```python
from build123d import *

# Parameters (mm, degrees)
BOSS_EXTRUDE1_DEPTH     = 42
CUT_EXTRUDE1_DEPTH      = 51.635955605
CUT_EXTRUDE1_DEPTH_BACK = 51.635955605
SKETCH2_R               = 1.125
CHAMFER1_SIZE           = 12
CHAMFER1_SIZE2          = 2.115923769
CHAMFER2_SIZE           = 12
CHAMFER2_SIZE2          = 2.115923769


with BuildPart() as part:
    # Sketch1 → Boss-Extrude1 (new body)
    with BuildSketch(Plane.XY):
        Polygon((0, 0), (0, 20), (4, 20), (4, 4), (20, 4), (20, 0), align=None)
    extrude(amount=BOSS_EXTRUDE1_DEPTH)

    # Sketch2 → Cut-Extrude1 (cut, two sides: drawn at the far end of the back side and taken through both)
    with BuildSketch(Plane(origin=(0, 0, 0), x_dir=(0, 0, -1), z_dir=(0.7071067811865475, -0.7071067811865477, 0)).offset(-CUT_EXTRUDE1_DEPTH_BACK)):
        with Locations(Location((-40, 2.828427125, 0), (0, 0, 90))):
            Circle(SKETCH2_R)
        with Locations(Location((-37.285714286, 2.828427125, 0), (0, 0, 90))):
            Circle(SKETCH2_R)
        with Locations(Location((-34.571428571, 2.828427125, 0), (0, 0, 90))):
            Circle(SKETCH2_R)
        with Locations(Location((-31.857142857, 2.828427125, 0), (0, 0, 90))):
            Circle(SKETCH2_R)
        with Locations(Location((-29.142857143, 2.828427125, 0), (0, 0, 90))):
            Circle(SKETCH2_R)
        with Locations(Location((-26.428571429, 2.828427125, 0), (0, 0, 90))):
            Circle(SKETCH2_R)
        with Locations(Location((-23.714285714, 2.828427125, 0), (0, 0, 90))):
            Circle(SKETCH2_R)
        with Locations(Location((-21, 2.828427125, 0), (0, 0, 90))):
            Circle(SKETCH2_R)
        with Locations(Location((-18.285714286, 2.828427125, 0), (0, 0, 90))):
            Circle(SKETCH2_R)
        with Locations(Location((-15.571428571, 2.828427125, 0), (0, 0, 90))):
            Circle(SKETCH2_R)
        with Locations(Location((-12.857142857, 2.828427125, 0), (0, 0, 90))):
            Circle(SKETCH2_R)
        with Locations(Location((-10.142857143, 2.828427125, 0), (0, 0, 90))):
            Circle(SKETCH2_R)
        with Locations(Location((-7.428571429, 2.828427125, 0), (0, 0, 90))):
            Circle(SKETCH2_R)
        with Locations(Location((-4.714285714, 2.828427125, 0), (0, 0, 90))):
            Circle(SKETCH2_R)
        with Locations(Location((-2, 2.828427125, 0), (0, 0, 90))):
            Circle(SKETCH2_R)
    extrude(amount=CUT_EXTRUDE1_DEPTH + CUT_EXTRUDE1_DEPTH_BACK, mode=Mode.SUBTRACT)

    # Chamfer1
    chamfer1_edges = [part.edges().sort_by_distance(p)[0] for p in [
        (20, 0, 21),
    ]]
    chamfer1_side = [part.faces().sort_by_distance(p)[0] for p in [
        (10.669713524, 0, 21),
    ]]
    chamfer(chamfer1_edges, length=CHAMFER1_SIZE, length2=CHAMFER1_SIZE2, reference=chamfer1_side[0])

    # Chamfer2
    chamfer2_edges = [part.edges().sort_by_distance(p)[0] for p in [
        (0, 20, 21),
    ]]
    chamfer2_side = [part.faces().sort_by_distance(p)[0] for p in [
        (0, 10.669713524, 21),
    ]]
    chamfer(chamfer2_edges, length=CHAMFER2_SIZE, length2=CHAMFER2_SIZE2, reference=chamfer2_side[0])


solid = part.part
```
CAD build for the part. Positions are in the model's coordinates, mm. Round coordinates to 2 decimals unless told otherwise and drop trailing zeros. Order: outer loops, then holes, each group sorted by start corner. A loop starts at its lowest first (then second) coordinate and runs counter-clockwise, first axis right, second up. Notation, with made-up numbers: (10, 54) - (36, 54) arc R34 ccw to (36, 92) - close; hole circle Ø8 at (61, -26). An arc over 180 degrees is marked (long way). Answer in a Markdown table with one row per item. Add a question column.
(1) Band-saw the part on D-D on y = 9.25. List the corners of the cut face in (x, z).
(2) Probe L1, parallel to Y at x = 7.75, z = 11; L2, parallel to Y at x = 9.5, z = 14. List the from-to ranges inside material, lowest first. Write a range as [from, to].
(3) Mould opens along Z. For faces 1 (the face through (3, 6, 0)), 2 (the face through (20, 3, 21)), 3 (the face through (2.7, 2.77, 12.43)) say: +Z half, -Z half, draft (parallel to the pull), parting line (faces both ways), or undercut.
(4) Drop flat-ended pins along their axis: pin 1 Ø6 at (y, z) = (13.5, 7.5) entering from +X; pin 2 Ø1.5 at (x, y) = (3.5, 17.5) entering from -Z; pin 3 Ø8 at (x, z) = (9.5, 24) entering from +Y; pin 4 Ø10 at (x, y) = (11.5, 15.5) entering from +Z. Give the stop position or say it passes through.
(5) Band-saw the part on B-B on z = 38. List the corners of the cut face in (x, y), and give its area (3 significant figures).
(6) Band-saw the part on C-C on x = 1.5. Count the separate pieces of the cut face and the enclosed holes in it, and give its area (3 significant figures).
(7) Band-saw the part on A-A on z = 21.5. List the corners of the cut face in (x, y).
Data:
| question | item | result |
|---|---|---|
| 1 | outline | (0.22, 0) - (4, 0) - (4, 42) - (0.22, 42) - close |
| 2 | L1 | y = [0, 4] |
| 2 | L2 | y = [0.26, 4] |
| 3 | face 1 | -Z half |
| 3 | face 2 | draft |
| 3 | face 3 | undercut |
| 4 | pin 1 | stops at x = 4 |
| 4 | pin 2 | stops at z = 0 |
| 4 | pin 3 | stops at y = 4 |
| 4 | pin 4 | passes through |
| 5 | outline | (0, 0) - (2.77, 0) - (0, 2.77) - close; (0, 5.23) - (5.23, 0) - (8, 0) - (20, 2.12) - (20, 4) - (4, 4) - (4, 20) - (2.12, 20) - (0, 8) - close |
| 5 | area | 109 mm^2 |
| 6 | separate pieces | 1 |
| 6 | enclosed holes | 15 |
| 6 | area | 609 mm^2 |
| 7 | outline | (0, 0) - (2.57, 0) - (0, 2.57) - close; (0, 5.43) - (5.43, 0) - (8, 0) - (20, 2.12) - (20, 4) - (4, 4) - (4, 20) - (2.12, 20) - (0, 8) - close |
